Work out the finished part from the listing and answer in its coordinate system (mm). Face numbers are marked on the shaded views. A direction names the side the tool comes from. Round coordinates to 2 decimals unless told otherwise and drop trailing zeros. Write each loop counter-clockwise with the first axis right and the second up, starting at its lowest first coordinate (ties: lowest second). Pieces come first, ordered by that corner, then holes. Notation, with made-up numbers: M 86,-33 L 122,-33 A14 cw 122,-25 Z; hole C 82,43 d11. An arc over 180 degrees is marked long. One line per item, written item: value. Start each with the question number.
Q1. The mould has two halves that part along X. Classify the marked faces 3, 4 and 5: released by +X, released by -X, zero draft, split by the parting line, or undercut.
Q2. Find section A-A (y = 265.5). Write down the section's boundary in (x, z).
Q3. Find section C-C (z = -7.5). Write down the section's boundary in (x, y).
Q4. Consider probe 1 along Z at (x, y) = (-9.5, 287); probe 2 along Z at (x, y) = (13.25, 163). Determine where each line is inside the solid, lowest interval first.
Q5. A tool of negligible diameter and unlimited length cuts with its end or side. For the marked faces 1 and 2, from which of +Z, -Z, +X, -X, +Y, -Y can it reach the whole face along a straight path? Write none if from no direction.
Q6. Find section B-B (x = 4). Write down the section's boundary in (y, z), and give its area (3 significant figures).
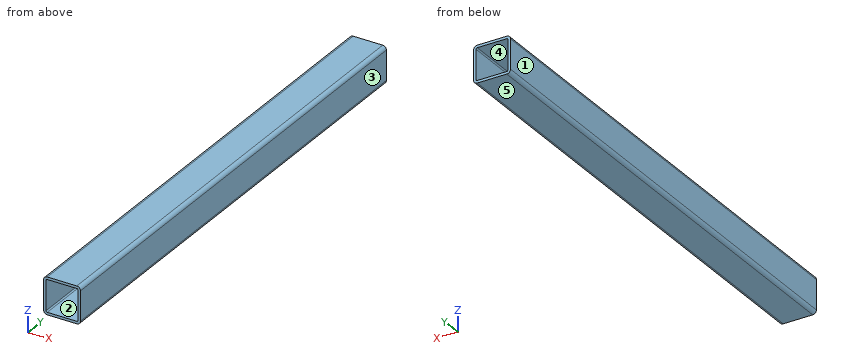
Autodesk Inventor part; units mm, degrees
ref_plane "YZ Plane" through (0, 0, 0) normal (1, 0, 0) x (0, 1, 0)
ref_plane "XZ Plane" through (0, 0, 0) normal (0, 1, 0) x (-1, 0, 0)
sketch "Sketch1" plane through (0, 0, 0) normal (0, 1, 0) x (-1, 0, 0)
  line L0 (-12, 14) -> (12, 14) construction
  line L1 (14, 12) -> (14, -12) construction
  line L2 (12, -14) -> (-12, -14) construction
  line L3 (-14, -12) -> (-14, 12) construction
  line L4 (-14, 14) -> (14, -14) construction
  line L5 (14, 14) -> (-14, -14) construction
  arc A0 (14, 12) -> (12, 14) centre (12, 12) ccw construction
  arc A1 (12, -14) -> (14, -12) centre (12, -12) ccw construction
  arc A2 (-14, -12) -> (-12, -14) centre (-12, -12) ccw construction
  arc A3 (-12, 14) -> (-14, 12) centre (-12, 12) ccw construction
  line L6 (-12, -15) -> (12, -15)
  arc A4 (12, -15) -> (15, -12) centre (12, -12) ccw
  line L7 (15, -12) -> (15, 12)
  arc A5 (15, 12) -> (12, 15) centre (12, 12) ccw
  line L8 (12, 15) -> (-12, 15)
  arc A6 (-12, 15) -> (-15, 12) centre (-12, 12) ccw
  line L9 (-15, 12) -> (-15, -12)
  arc A7 (-15, -12) -> (-12, -15) centre (-12, -12) ccw
  line L10 (13, -12) -> (13, 12)
  arc A8 (13, 12) -> (12, 13) centre (12, 12) ccw
  line L11 (12, 13) -> (-12, 13)
  arc A9 (-12, 13) -> (-13, 12) centre (-12, 12) ccw
  line L12 (-13, 12) -> (-13, -12)
  arc A10 (-13, -12) -> (-12, -13) centre (-12, -12) ccw
  line L13 (-12, -13) -> (12, -13)
  arc A11 (12, -13) -> (13, -12) centre (12, -12) ccw
  point P0 (0, 0)
  point P1 (0, 0)
  point P2 (0, 0)
  dimension "d10" = 2
  dimension "depth" = 30
  dimension "width" = 30
  dimension "thickness" = 2
extrude "Extrusion1" add sketch "Sketch1" along normal blind 400
ref_plane "Work Plane1" through (0, 200, 0) normal (0, -1, 0) x (1, 0, 0)
equation "\"d10\" = thickness"
properties part number "podest duzy profil 8" material "Steel"
The answers:
1. face 3: released by +X
1. face 4: undercut
1. face 5: zero draft
2. outline: M -15,-12 A3 ccw -12,-15 L 12,-15 A3 ccw 15,-12 L 15,12 A3 ccw 12,15 L -12,15 A3 ccw -15,12 Z; hole M -13,-12 A1 ccw -12,-13 L 12,-13 A1 ccw 13,-12 L 13,12 A1 ccw 12,13 L -12,13 A1 ccw -13,12 Z
3. outline: M -15,0 L -13,0 L -13,400 L -15,400 Z; M 13,0 L 15,0 L 15,400 L 13,400 Z
4. probe 1: -15 to -13, 13 to 15
4. probe 2: -14.73 to 14.73
5. face 1: +Z, -Z, -X, +Y, -Y
5. face 2: +Y, -Y
6. outline: M 0,-15 L 400,-15 L 400,-13 L 0,-13 Z; M 0,13 L 400,13 L 400,15 L 0,15 Z
6. area: 1,600 mm2
